Build history of the part. All positions in model axes, mm. A direction names the side the tool comes from. Round coordinates to 2 decimals unless told otherwise and drop trailing zeros. Order: outer loops, then holes, each group sorted by start corner. A loop starts at its lowest first (then second) coordinate and runs counter-clockwise, first axis right, second up. Notation, with made-up numbers: (-6.5, 68) -> (13.5, 68) arc R15 cw to (13.5, 97) -> close; hole circle Ø2 at (32.25, 58.5). An arc over 180 degrees is marked (long way). Write item = value, one per line.
from build123d import *

# Parameters (mm, degrees)
SKETCH_1_W               = 20
SKETCH_1_H               = 15
SKETCH_1_W_2             = 14
SKETCH_1_H_2             = 9
EXTRUDE_1_DEPTH          = 16.5
SKETCH_2_W               = 6.10870136
SKETCH_2_H               = 6
CUT_EXTRUDE_1_DEPTH      = 18
CUT_EXTRUDE_1_DEPTH_BACK = 4
CUT_EXTRUDE_2_DEPTH      = 13
CUT_EXTRUDE_2_DEPTH_BACK = 4
SKETCH_5_R               = 3.5
CUT_EXTRUDE_3_DEPTH      = 18
CUT_EXTRUDE_3_DEPTH_BACK = 4
SKETCH_6_W               = 3
SKETCH_6_H               = 4
EXTRUDE_2_DEPTH          = 4
FILLET_1_R               = 0.3
FILLET_2_R               = 0.3


with BuildPart() as part:
    # Эскиз1 → Бобышка-Вытянуть1 (new body)
    with BuildSketch(Plane(origin=(0, 0, 0), x_dir=(1, 0, 0), z_dir=(0, 1, 0))):
        Rectangle(SKETCH_1_W, SKETCH_1_H)
        Rectangle(SKETCH_1_W_2, SKETCH_1_H_2, mode=Mode.SUBTRACT)
    extrude(amount=-EXTRUDE_1_DEPTH)

    # Эскиз2 → Вырез-Вытянуть1 (cut, two sides)
    with BuildSketch(Plane.ZY.offset(-7)) as cut_extrude_1_sk:
        with Locations((0, -4.4)):
            Rectangle(SKETCH_2_W, SKETCH_2_H)
    extrude(amount=CUT_EXTRUDE_1_DEPTH, mode=Mode.SUBTRACT)
    extrude(cut_extrude_1_sk.sketch, amount=-CUT_EXTRUDE_1_DEPTH_BACK, mode=Mode.SUBTRACT)

    # Эскиз4 → Вырез-Вытянуть2 (cut, two sides)
    with BuildSketch(Plane(origin=(0, 0, 4.5), x_dir=(-1, 0, 0), z_dir=(0, 0, -1))) as cut_extrude_2_sk:
        with BuildLine():
            Line((-1, -13), (1, -13))
            ThreePointArc((1, -13), (4.5, -16.5), (1, -20))
            Line((1, -20), (-1, -20))
            ThreePointArc((-1, -20), (-4.5, -16.5), (-1, -13))
        make_face()
    extrude(amount=CUT_EXTRUDE_2_DEPTH, mode=Mode.SUBTRACT)
    extrude(cut_extrude_2_sk.sketch, amount=-CUT_EXTRUDE_2_DEPTH_BACK, mode=Mode.SUBTRACT)

    # Эскиз5 → Вырез-Вытянуть3 (cut, two sides)
    with BuildSketch(Plane(origin=(-7, 0, 0), x_dir=(0, 0, -1), z_dir=(1, 0, 0))) as cut_extrude_3_sk:
        with Locations((0, -16.5)):
            Circle(SKETCH_5_R)
    extrude(amount=CUT_EXTRUDE_3_DEPTH, mode=Mode.SUBTRACT)
    extrude(cut_extrude_3_sk.sketch, amount=-CUT_EXTRUDE_3_DEPTH_BACK, mode=Mode.SUBTRACT)

    # Эскиз6 → Бобышка-Вытянуть2 (add)
    with BuildSketch(Plane.XZ.offset(16.5)):
        with Locations((-8.5, -5.5)):
            Rectangle(SKETCH_6_W, SKETCH_6_H)
        with Locations((-8.5, 5.5)):
            Rectangle(SKETCH_6_W, SKETCH_6_H)
        with Locations((8.5, 5.5)):
            Rectangle(SKETCH_6_W, SKETCH_6_H)
        with Locations((8.5, -5.5)):
            Rectangle(SKETCH_6_W, SKETCH_6_H)
    extrude(amount=EXTRUDE_2_DEPTH)

    # Скругление1
    fillet_1_edges = [part.edges().sort_by_distance(p)[0] for p in [
        (-10, -10.25, -7.5),
        (10, -10.25, -7.5),
        (10, -10.25, 7.5),
        (-10, -10.25, 7.5),
    ]]
    fillet(fillet_1_edges, radius=FILLET_1_R)

    # Скругление2
    fillet_2_edges = [part.edges().sort_by_distance(p)[0] for p in [
        (-10, -18.5, -3.5),
        (-7, -18.5, -7.5),
        (-7, -18.5, -3.5),
        (-7, -18.5, 3.5),
        (-7, -18.5, 7.5),
        (-10, -18.5, 3.5),
        (7, -18.5, 7.5),
        (7, -18.5, 3.5),
        (10, -18.5, 3.5),
        (7, -18.5, -3.5),
        (7, -18.5, -7.5),
        (10, -18.5, -3.5),
        (-3.474873734, -14.025126266, 4.5),
        (0, -13, 4.5),
        (3.474873734, -14.025126266, 4.5),
        (0, -13, 7.5),
        (3.474873734, -14.025126266, -7.5),
        (-3.474873734, -14.025126266, -7.5),
        (3.474873734, -14.025126266, -4.5),
        (3.474873734, -14.025126266, 7.5),
        (0, -13, -7.5),
        (-3.474873734, -14.025126266, -4.5),
        (-3.474873734, -14.025126266, 7.5),
        (0, -13, -4.5),
        (7, -13, 0),
        (10, -13, 0),
        (-10, -13, 0),
        (-7, -13, 0),
    ]]
    fillet(fillet_2_edges, radius=FILLET_2_R)


solid = part.part
Q1. Cut at C-C, the plane x = 6.5. List the corners of the cut face in (y, z), and give its area (3 significant figures).
Check values:
outline = (-16.5, -7.5) -> (0, -7.5) -> (0, -4.5) -> (-16.5, -4.5) -> close; (-16.5, 4.5) -> (0, 4.5) -> (0, 7.5) -> (-16.5, 7.5) -> close
area = 99.0 mm²
Q2. Cut at B-B, the plane z = 0. List the corners of the cut face in (x, y).
Check values:
outline = (-10, -12.7) arc R0.3 ccw to (-9.7, -13) -> (-7.3, -13) arc R0.3 ccw to (-7, -12.7) -> (-7, -7.4) -> (-10, -7.4) -> close; (-10, -1.4) -> (-7, -1.4) -> (-7, 0) -> (-10, 0) -> close; (7, -12.7) arc R0.3 ccw to (7.3, -13) -> (9.7, -13) arc R0.3 ccw to (10, -12.7) -> (10, -7.4) -> (7, -7.4) -> close; (7, -1.4) -> (10, -1.4) -> (10, 0) -> (7, 0) -> close
Q3. Cut at D-D, the plane z = -5.25. List the corners of the cut face in (x, y), and give its area (3 significant figures).
Check values:
outline = (-10, -20.5) -> (-7, -20.5) -> (-7, -16.5) -> (-4.5, -16.5) arc R3.5 cw to (-1, -13) -> (1, -13) arc R3.5 cw to (4.5, -16.5) -> (7, -16.5) -> (7, -20.5) -> (10, -20.5) -> (10, 0) -> (-10, 0) -> close
area = 328 mm²
Q4. Which spindle directions (+Z, -Z, +X, -X, +Y, -Y) get a long thin tool onto all of the face, cutting with end or side? Do faces 4 (the face through (-3.45, -14, 5.98)), 5 (the face through (8, -7.4, 0)), 6 (the face through (8, -18, -3.5)), 7 (the face through (7, -10, 0)), 8 (the face through (-9, -20.5, 6)). Say none if no direction does.
Check values:
face_4 = +Z, -Z, -Y
face_5 = +X, -X
face_6 = +X, -X, -Y
face_7 = -Y
face_8 = +Z, -Z, +X, -X, -Y
Q5. Mould opens along Y. For faces 1 (the face through (3.5, -14.05, -5.98)), 2 (the face through (8, -4, -3.054)), 3 (the face through (-9, -18, -3.5)) say: released by +Y, released by -Y, zero draft, split by the parting line, or undercut.
Check values:
face_1 = released by -Y
face_2 = undercut
face_3 = zero draft
Q6. Cut at A-A, the plane y = -2. List the corners of the cut face in (x, z).
Check values:
outline = (-10, -7.2) arc R0.3 ccw to (-9.7, -7.5) -> (9.7, -7.5) arc R0.3 ccw to (10, -7.2) -> (10, -3.05) -> (7, -3.05) -> (7, -4.5) -> (-7, -4.5) -> (-7, -3.05) -> (-10, -3.05) -> close; (-10, 3.05) -> (-7, 3.05) -> (-7, 4.5) -> (7, 4.5) -> (7, 3.05) -> (10, 3.05) -> (10, 7.2) arc R0.3 ccw to (9.7, 7.5) -> (-9.7, 7.5) arc R0.3 ccw to (-10, 7.2) -> close
Q7. Probe probe 1 along X at (y, z) = (-3, -3.75); probe 2 along Z at (x, y) = (-3, -10); probe 3 along X at (y, z) = (-16.25, -4.75). List the from-to ranges inside material, lowest first.
Check values:
probe_1 = -10 to -7, 7 to 10
probe_2 = -7.5 to -4.5, 4.5 to 7.5
probe_3 = -10 to -4.5, 4.5 to 10
Q8. Flat gauge pins, fed straight in: pin 1 (0.8 mm diameter, centred on x = -6, z = -6.5, fed in from -Y); pin 2 (1.5 mm diameter, centred on y = -17, z = -1.5, fed in from +X); pin 3 (1 mm diameter, centred on x = -1, z = -5.5, fed in from -Y); pin 4 (3.5 mm diameter, centred on x = 8, z = 0, fed in from -Y). Where does each tip first touch, or does it go through?
Check values:
pin_1 = -16.5
pin_2 = through
pin_3 = -13.04
pin_4 = -13.47
